```python
from build123d import *

# Parameters (mm, degrees)
BOSS_EXTRUDE1_DEPTH = 5.08
FILLET1_R           = 20
SKETCH2_W           = 5
SKETCH2_H           = 7
SKETCH2_W_2         = 10
SKETCH2_H_2         = 5.08
CUT_EXTRUDE1_DEPTH  = 6.08


with BuildPart() as part:
    # Sketch1 → Boss-Extrude1 (new body)
    with BuildSketch(Plane.XY):
        Polygon((-100, 5.08), (-100, 10.16), (100, 10.16), (100, -10.16), (-100, -10.16), (-100, -5.08), (-120, -5.08), (-120, 5.08), align=None)
    extrude(amount=BOSS_EXTRUDE1_DEPTH)

    # Fillet1
    fillet1_edges = [part.edges().sort_by_distance(p)[0] for p in [
        (100, -10.16, 2.54),
    ]]
    fillet(fillet1_edges, radius=FILLET1_R)

    # Sketch2 → Cut-Extrude1 (cut, through all)
    with BuildSketch(Plane.XY.offset(5.08)):
        with Locations((-15.04, -6.66)):
            Rectangle(SKETCH2_W, SKETCH2_H)
        with Locations((84.96, -6.66)):
            Rectangle(SKETCH2_W, SKETCH2_H)
        with Locations((-65, 2.54)):
            Rectangle(SKETCH2_W_2, SKETCH2_H_2)
        with Locations((-15, 2.54)):
            Rectangle(SKETCH2_W_2, SKETCH2_H_2)
        with Locations((35, 2.54)):
            Rectangle(SKETCH2_W_2, SKETCH2_H_2)
        with Locations((85, 2.54)):
            Rectangle(SKETCH2_W_2, SKETCH2_H_2)
    extrude(amount=-CUT_EXTRUDE1_DEPTH, mode=Mode.SUBTRACT)


solid = part.part
```
Build history of the part. All positions in model axes, mm. A direction names the side the tool comes from. Coordinates: 2 decimals unless noted, no trailing zeros. Write each loop counter-clockwise with the first axis right and the second up, starting at its lowest first coordinate (ties: lowest second). Pieces come first, ordered by that corner, then holes.
1. Drill centre lines: probe 1 along X at (y, z) = (-3.5, 2.4); probe 2 along X at (y, z) = (4.25, 1.5); probe 3 along X at (y, z) = (1.5, 2.7). Where is each one in solid material? Low to high.
Answer block:
probe 1: x = -120 to -17.54, -12.54 to 82.46, 87.46 to 94.9
probe 2: x = -120 to -70, -60 to -20, -10 to 30, 40 to 80, 90 to 99.2
probe 3: x = -120 to -70, -60 to -20, -10 to 30, 40 to 80, 90 to 98.18
2. Band-saw the part on A-A, the plane x = 35. Give the cut face in (y, z), and give its area (3 significant figures).
Answer block:
outline: (-10.16, 0) - (0, 0) - (0, 5.08) - (-10.16, 5.08) - close; (5.08, 0) - (10.16, 0) - (10.16, 5.08) - (5.08, 5.08) - close
area: 77.4 mm2
3. Drop flat-ended pins along their axis: pin 1 (2.5 mm diameter, centred on x = -14, z = 2.5, fed in from -Y); pin 2 (2.5 mm diameter, centred on y = 4, z = 2, fed in from +X). Give the stop position or say it passes through.
Answer block:
pin 1: stops at y = -3.16
pin 2: stops at x = 99.47
4. Band-saw the part on B-B, the plane z = 2.65. Give the number of separate pieces and of enclosed holes in the cut face, and give its area (3 significant figures).
Answer block:
separate pieces: 1
enclosed holes: 4
area: 3,910 mm2
5. 3-axis set-ups, long thin cutter, end or side, ignore diameter. For faces 1 (the flat face through (-100, 8, 3)), 2 (the flat face through (-110, -5.08, 3)), 3 (the flat face through (-15, 0, 3)): which of +Z, -Z, +X, -X, +Y, -Y reach the whole face in a straight line?
Answer block:
face 1: +Z, -Z, -X, +Y
face 2: +Z, -Z, -X, -Y
face 3: +Z, -Z
6. Pull direction Y, two halves, no side cores. Call faces 4 (the flat face through (-1, 10.16, 3)), 5 (the flat face through (90, 3, 3)), 6 (the flat face through (-8, 0, 0)): released by +Y, released by -Y, zero draft, split by the parting line, or undercut.
Answer block:
face 4: released by +Y
face 5: undercut
face 6: zero draft
